Could you check a few things on this model? Use its own coordinates, in mm. A direction names the side the tool comes from. Give positions to 0.01 mm unless a question says otherwise; leave off trailing zeros. Write each loop counter-clockwise with the first axis right and the second up, starting at its lowest first coordinate (ties: lowest second). Pieces come first, ordered by that corner, then holes. Notation, with made-up numbers: M 9,31.5 L 43,31.5 A22 cw 43,66.5 Z; hole C 47,-21 d3. An arc over 180 degrees is marked long. Write each question's results on one line, items separated by ' | '. Start each with the question number.
from build123d import *

# Parameters (mm, degrees)
SKETCH1_R           = 2
SKETCH1_R_2         = 3.125
SKETCH1_R_3         = 1.7
BOSS_EXTRUDE1_DEPTH = 10
FILLET2_R           = 3
FILLET1_R           = 2
SKETCH1_4_R         = 3.125
CUT_EXTRUDE3_DEPTH  = 5.07
SKETCH1_7_R         = 1.7
CUT_EXTRUDE6_DEPTH  = 10
CUT_EXTRUDE5_DEPTH  = 3
SKETCH1_5_R         = 2
CUT_EXTRUDE4_DEPTH  = 2.48
SKETCH4_R           = 1.5
CUT_EXTRUDE7_DEPTH  = 10
SKETCH5_R           = 2.725
CUT_EXTRUDE8_DEPTH  = 2.8
BOSS_EXTRUDE2_DEPTH = 10
BOSS_EXTRUDE3_DEPTH = 50
FILLET13_R          = 5
CUT_EXTRUDE14_DEPTH = 15
SKETCH10_W          = 8
SKETCH10_H          = 6
CUT_EXTRUDE12_DEPTH = 40
FILLET12_R          = 2
FILLET14_R          = 2
CUT_EXTRUDE17_DEPTH = 20
SKETCH19_R          = 1.5
CUT_EXTRUDE18_DEPTH = 4


with BuildPart() as part:
    # Sketch1 → Boss-Extrude1 (new body)
    with BuildSketch(Plane(origin=(0, 0, 0), x_dir=(1, 0, 0), z_dir=(0, 1, 0))):
        with BuildLine():
            ThreePointArc((-11.409245094, 8.977987014), (-9.849239736, 9.28), (-8.289234378, 8.977987014))
            ThreePointArc((-8.289234378, 8.977987014), (-5.835653376, 8.254222737), (-3.289234378, 8.01))
            Line((-3.289234378, 8.01), (38.12, 8.01))
            Line((38.12, 8.01), (38.12, -3.81))
            Line((38.12, -3.81), (28.478275237, -3.81))
            Line((28.478275237, -3.81), (26.178275237, 0))
            Line((26.178275237, 0), (-26.178275237, 0))
            Line((-26.178275237, 0), (-28.478275237, -3.81))
            Line((-28.478275237, -3.81), (-38.12, -3.81))
            Line((-38.12, -3.81), (-38.12, 8.01))
            Line((-38.12, 8.01), (-16.409245094, 8.01))
            ThreePointArc((-16.409245094, 8.01), (-13.862826096, 8.254222737), (-11.409245094, 8.977987014))
        make_face()
        with Locations((22, 4.005)):
            Circle(SKETCH1_R, mode=Mode.SUBTRACT)
        with Locations((-22, 4.005)):
            Circle(SKETCH1_R, mode=Mode.SUBTRACT)
        with Locations((-32.12, 1.98)):
            Circle(SKETCH1_R_2, mode=Mode.SUBTRACT)
        with Locations((32.12, 1.98)):
            Circle(SKETCH1_R_2, mode=Mode.SUBTRACT)
        with Locations((-9.849239736, 5.1)):
            Circle(SKETCH1_R_3, mode=Mode.SUBTRACT)
        with BuildLine():
            ThreePointArc((11.912105026, 2.53), (14.127105026, 4.745), (11.912105026, 6.96))
            Line((11.912105026, 6.96), (5.992105026, 6.96))
            ThreePointArc((5.992105026, 6.96), (3.777105026, 4.745), (5.992105026, 2.53))
            Line((5.992105026, 2.53), (11.912105026, 2.53))
        make_face(mode=Mode.SUBTRACT)
        with Locations((-22, 4.005)):
            Circle(SKETCH1_R)
        with Locations((-9.849239736, 5.1)):
            Circle(SKETCH1_R_3)
        with Locations((-32.12, 1.98)):
            Circle(SKETCH1_R_2)
        with BuildLine():
            Line((5.992105026, 2.53), (11.912105026, 2.53))
            ThreePointArc((11.912105026, 2.53), (14.127105026, 4.745), (11.912105026, 6.96))
            Line((11.912105026, 6.96), (5.992105026, 6.96))
            ThreePointArc((5.992105026, 6.96), (3.777105026, 4.745), (5.992105026, 2.53))
        make_face()
        with Locations((22, 4.005)):
            Circle(SKETCH1_R)
        with Locations((32.12, 1.98)):
            Circle(SKETCH1_R_2)
    extrude(amount=-BOSS_EXTRUDE1_DEPTH)

    # Fillet2
    fillet2_edges = [part.edges().sort_by_distance(p)[0] for p in [
        (28.478275237, -5, 3.81),
        (-28.478275237, -5, 3.81),
    ]]
    fillet(fillet2_edges, radius=FILLET2_R)

    # Fillet1
    fillet1_edges = [part.edges().sort_by_distance(p)[0] for p in [
        (26.178275237, -5, 0),
        (-26.178275237, -5, 0),
    ]]
    fillet(fillet1_edges, radius=FILLET1_R)

    # Sketch1_4 → Cut-Extrude3 (cut)
    with BuildSketch(Plane(origin=(0, 0, 0), x_dir=(1, 0, 0), z_dir=(0, 1, 0))):
        with Locations(Location((32.12, 1.98, 0), (0, 0, 270))):
            Circle(SKETCH1_4_R)
        with Locations(Location((-32.12, 1.98, 0), (0, 0, 270))):
            Circle(SKETCH1_4_R)
    extrude(amount=-CUT_EXTRUDE3_DEPTH, mode=Mode.SUBTRACT)

    # Sketch1_7 → Cut-Extrude6 (cut)
    with BuildSketch(Plane(origin=(0, 0, 0), x_dir=(1, 0, 0), z_dir=(0, 1, 0))):
        with Locations(Location((-9.849239736, 5.1, 0), (0, 0, 270))):
            Circle(SKETCH1_7_R)
    extrude(amount=-CUT_EXTRUDE6_DEPTH, mode=Mode.SUBTRACT)

    # Sketch1_6 → Cut-Extrude5 (cut)
    with BuildSketch(Plane(origin=(0, 0, 0), x_dir=(1, 0, 0), z_dir=(0, 1, 0))):
        with BuildLine():
            Line((5.992105026, 2.53), (11.912105026, 2.53))
            ThreePointArc((11.912105026, 2.53), (14.127105026, 4.745), (11.912105026, 6.96))
            Line((11.912105026, 6.96), (5.992105026, 6.96))
            ThreePointArc((5.992105026, 6.96), (3.777105026, 4.745), (5.992105026, 2.53))
        make_face()
    extrude(amount=-CUT_EXTRUDE5_DEPTH, mode=Mode.SUBTRACT)

    # Sketch1_5 → Cut-Extrude4 (cut)
    with BuildSketch(Plane(origin=(0, 0, 0), x_dir=(1, 0, 0), z_dir=(0, 1, 0))):
        with Locations(Location((-22, 4.005, 0), (0, 0, 270))):
            Circle(SKETCH1_5_R)
        with Locations(Location((22, 4.005, 0), (0, 0, 270))):
            Circle(SKETCH1_5_R)
    extrude(amount=-CUT_EXTRUDE4_DEPTH, mode=Mode.SUBTRACT)

    # Sketch4 → Cut-Extrude7 (cut)
    with BuildSketch(Plane(origin=(0, 0, 0), x_dir=(1, 0, 0), z_dir=(0, 1, 0))):
        with Locations(Location((-22, 4.005, 0), (0, 0, 270))):
            Circle(SKETCH4_R)
        with Locations(Location((22, 4.005, 0), (0, 0, 270))):
            Circle(SKETCH4_R)
    extrude(amount=-CUT_EXTRUDE7_DEPTH, mode=Mode.SUBTRACT)

    # Sketch5 → Cut-Extrude8 (cut)
    with BuildSketch(Plane.XZ.offset(10)):
        with Locations(Location((22, -4.005, 0), (0, 0, 270))):
            Circle(SKETCH5_R)
        with Locations(Location((-22, -4.005, 0), (0, 0, 90))):
            Circle(SKETCH5_R)
    extrude(amount=-CUT_EXTRUDE8_DEPTH, mode=Mode.SUBTRACT)

    # Sketch6 → Boss-Extrude2 (add)
    with BuildSketch(Plane(origin=(0, 0, 0), x_dir=(1, 0, 0), z_dir=(0, 1, 0))):
        with BuildLine():
            Line((-38.12, 8.01), (-38.12, 18.01))
            Line((-38.12, 18.01), (38.12, 18.01))
            Line((38.12, 18.01), (38.12, 8.01))
            Line((38.12, 8.01), (-3.289234378, 8.01))
            ThreePointArc((-3.289234378, 8.01), (-5.835653376, 8.254222737), (-8.289234378, 8.977987014))
            ThreePointArc((-8.289234378, 8.977987014), (-9.849239736, 9.28), (-11.409245094, 8.977987014))
            ThreePointArc((-11.409245094, 8.977987014), (-13.862826096, 8.254222737), (-16.409245094, 8.01))
            Line((-16.409245094, 8.01), (-38.12, 8.01))
        make_face()
    extrude(amount=-BOSS_EXTRUDE2_DEPTH)

    # Sketch8 → Boss-Extrude3 (add)
    with BuildSketch(Plane.XZ.offset(10)):
        with BuildLine():
            Line((18.950546011, 0), (-18.950546011, 0))
            Line((-18.950546011, 0), (-18.950546011, -4.005))
            ThreePointArc((-18.950546011, -4.005), (-22, -7.054453989), (-25.049453989, -4.005))
            Line((-25.049453989, -4.005), (-25.049453989, 0))
            ThreePointArc((-25.049453989, 0), (-26.032503369, 0.25827272), (-26.761657912, 0.966386084))
            Line((-26.761657912, 0.966386084), (-27.603201224, 2.360420875))
            ThreePointArc((-27.603201224, 2.360420875), (-28.696933037, 3.422590919), (-30.171507108, 3.81))
            Line((-30.171507108, 3.81), (-38.12, 3.81))
            Line((-38.12, 3.81), (-38.12, -18.01))
            Line((-38.12, -18.01), (38.12, -18.01))
            Line((38.12, -18.01), (38.12, 3.81))
            Line((38.12, 3.81), (30.171507108, 3.81))
            ThreePointArc((30.171507108, 3.81), (28.696933037, 3.422590919), (27.603201224, 2.360420875))
            Line((27.603201224, 2.360420875), (26.761657912, 0.966386084))
            ThreePointArc((26.761657912, 0.966386084), (26.032503369, 0.25827272), (25.049453989, 0))
            Line((25.049453989, 0), (25.049453989, -4.005))
            ThreePointArc((25.049453989, -4.005), (22, -7.054453989), (18.950546011, -4.005))
            Line((18.950546011, -4.005), (18.950546011, 0))
        make_face()
    extrude(amount=BOSS_EXTRUDE3_DEPTH)

    # Fillet13
    fillet13_edges = [part.edges().sort_by_distance(p)[0] for p in [
        (-38.12, -30, -18.01),
    ]]
    fillet(fillet13_edges, radius=FILLET13_R)

    # Sketch8_3 → Cut-Extrude14 (cut)
    with BuildSketch(Plane.XZ.offset(10)):
        with BuildLine():
            Line((-4.849239736, 0), (-4.849239736, -5.1))
            ThreePointArc((-4.849239736, -5.1), (-9.849239736, -10.1), (-14.849239736, -5.1))
            Line((-14.849239736, -5.1), (-14.849239736, 0))
            Line((-14.849239736, 0), (-4.849239736, 0))
        make_face()
    extrude(amount=CUT_EXTRUDE14_DEPTH, mode=Mode.SUBTRACT)

    # Sketch10 → Cut-Extrude12 (cut)
    with BuildSketch(Plane(origin=(38.12, 0, 0), x_dir=(0, 0, -1), z_dir=(1, 0, 0))):
        with Locations((12.01, -3)):
            Rectangle(SKETCH10_W, SKETCH10_H)
    extrude(amount=-CUT_EXTRUDE12_DEPTH, mode=Mode.SUBTRACT)

    # Fillet12
    fillet12_edges = [part.edges().sort_by_distance(p)[0] for p in [
        (-4.849239736, -17.5, 0),
        (-14.849239736, -17.5, 0),
    ]]
    fillet(fillet12_edges, radius=FILLET12_R)

    # Fillet14
    fillet14_edges = [part.edges().sort_by_distance(p)[0] for p in [
        (-1.88, -3, -16.01),
        (18.12, -6, -16.01),
        (-1.88, -3, -8.01),
    ]]
    fillet(fillet14_edges, radius=FILLET14_R)

    # Sketch18 → Cut-Extrude17 (cut)
    with BuildSketch(Plane.XZ.offset(60)):
        Polygon((-10, 0), (-10, -3), (-12.5, -3), (-12.5, -6), (12.5, -6), (12.5, -3), (10, -3), (10, 0), align=None)
    extrude(amount=-CUT_EXTRUDE17_DEPTH, mode=Mode.SUBTRACT)

    # Sketch19 → Cut-Extrude18 (cut)
    with BuildSketch(Plane.XY.offset(-6)):
        with Locations((0, -44)):
            Circle(SKETCH19_R)
    extrude(amount=-CUT_EXTRUDE18_DEPTH, mode=Mode.SUBTRACT)


solid = part.part
Q1. For faces 1 (the face through (-20.8, -7.2, -2.8)), 2 (the face through (-10, -25, -5)), 3 (the face through (-10, -50, -1)), which set-ups out of +Z, -Z, +X, -X, +Y, -Y let a thin tool reach every point of the face, with its end or its side?
Q2. If we section it at C-C (x = -32.12): Please give me the cut outline in (y, z) (3 decimals).
Q3. If we mould it in two halves opening along Y, with no side actions, what happens to faces 4 (the face through (-29.02, -2.5, -2.39)), 5 (the face through (18, -6, -11)), 6 (the face through (0, -44, -10)), 7 (the face through (-0.325, -45.464, -7.972))? For each: pulls with the +Y half, pulls with the -Y half, needs draft (parallel to the pull), parting line crosses it, or undercut.
Q4. If we section it at D-D (y = -23): Please give me the cut outline in (x, z) (1 decimal).
Q5. I'm going to push flat-ended pins straight in: P1, Ø4.5, axis at y = -3, z = -12.5, coming from the +X side; P2, Ø3, axis at x = 26.5, y = -2.5, coming from the +Z side; P3, Ø4.5, axis at x = 21.5, z = -3, coming from the -Y side; P4, Ø1, axis at x = -15.5, z = 1.5, coming from the -Y side. Where does each tip first touch, or does it pass through?
Q6. Please list where these lines run through material, in increasing order: line 1 (X direction, y = -2.6, z = -1.98) (3 decimals); line 2 (X direction, y = -42.5, z = -1); line 3 (Y direction, x = 19, z = -1.5). Write a range as [from, to].
Q7. If we section it at A-A (x = 22): Please give me the cut outline in (y, z) (3 decimals).
Determined:
1) face 1: -Y | face 2: +Z | face 3: +Z, -Y
2) outline: M -60,-18.01 L 0,-18.01 L 0,-5.105 L -5.07,-5.105 L -5.07,1.145 L 0,1.145 L 0,3.81 L -60,3.81 Z
3) face 4: needs draft | face 5: pulls with the +Y half | face 6: undercut | face 7: undercut
4) outline: M -38.1,-13 A5 ccw -33.1,-18 L 38.1,-18 L 38.1,3.8 L 30.2,3.8 A3 ccw 27.6,2.4 L 26.8,1 A2 cw 25,0 L 25,-4 A3 cw 19,-4 L 19,0 L -2.8,0 A2 ccw -4.8,-2 L -4.8,-5.1 A5 cw -14.8,-5.1 L -14.8,-2 A2 ccw -16.8,0 L -19,0 L -19,-4 A3 cw -25,-4 L -25,0 A2 cw -26.8,1 L -27.6,2.4 A3 ccw -30.2,3.8 L -38.1,3.8 Z
5) P1: stops at x = -1.74 | P2: stops at z = 2.88 | P3: stops at y = -10 | P4: passes through
6) line 1: x = [-38.12, -35.245], [-28.995, 28.995], [35.245, 38.12] | line 2: x = [-38.12, -25.05], [-18.95, -10], [10, 18.95], [25.05, 38.12] | line 3: y = [-10, 0]
7) outline: M -60,-18.01 L 0,-18.01 L 0,-16.01 L -4,-16.01 A2 cw -6,-14.01 L -6,-8.01 L 0,-8.01 L 0,-6.005 L -2.48,-6.005 L -2.48,-5.505 L -7.2,-5.505 L -7.2,-6.73 L -10,-6.73 L -10,-7.054 L -60,-7.054 Z; M -10,-1.28 L -7.2,-1.28 L -7.2,-2.505 L -2.48,-2.505 L -2.48,-2.005 L 0,-2.005 L 0,0 L -10,0 Z
